Could you check a few things on this model? Use its own coordinates, in mm. Face numbers are marked on the shaded views. A direction names the side the tool comes from. Coordinates: 2 decimals unless noted, no trailing zeros. Order: outer loops, then holes, each group sorted by start corner. A loop starts at its lowest first (then second) coordinate and runs counter-clockwise, first axis right, second up. Notation, with made-up numbers: (28.5, 59) - (58.5, 59) arc R5 cw to (58.5, 66) - close; hole circle Ø1 at (18.25, -23). An arc over 180 degrees is marked (long way). Answer as CSV lines item,"result". Start each with the question number.
1. I want a section at C-C, the plane y = 0. Count the separate pieces of the cut face and the enclosed holes in it, and give its area (3 significant figures).
2. I want a section at D-D, the plane x = 9. List the corners of the cut face in (y, z) for me, and give its area (3 significant figures).
3. I need wall thicknesses on probe 1 along Z at (x, y) = (5, 4); probe 2 along Z at (x, y) = (2, 7); probe 3 along Y at (x, z) = (0.5, -1). Which ranges of each line are inside material? Lowest first, please.
4. Thinking about a two-plate mould opening in Y: for the marked faces 1, 2 and 3, which applies, released by +Y, released by -Y, zero draft, split by the parting line, or undercut?
5. I want a section at A-A, the plane x = 14.5. List the corners of the cut face in (y, z) for me, and give its area (3 significant figures).
6. For pin 1 (1.5 mm diameter, centred on x = 13, y = -12.5, fed in from -Z); pin 2 (2 mm diameter, centred on x = -10.5, z = 1.5, fed in from -Y); pin 3 (4 mm diameter, centred on x = 5.5, z = -0.5, fed in from -Y); pin 4 (3 mm diameter, centred on x = -9.9, y = -9.9, fed in from +Z), each with a flat end and sliding along its axis, tell me the tip position at first contact or that it passes through.
7. For the marked faces 4, 5 and 6, which set-ups out of +Z, -Z, +X, -X, +Y, -Y let a thin tool reach every point of the face, with its end or its side?
from build123d import *

# Parameters (mm, degrees)
SKETCH_1_R          = 17.5
EXTRUDE_1_DEPTH     = 2
SKETCH_2_R          = 7
EXTRUDE_2_DEPTH     = 7
SKETCH_3_R          = 17.5
EXTRUDE_3_DEPTH     = 2
SKETCH_4_W          = 5
SKETCH_4_H          = 5
CUT_EXTRUDE_1_DEPTH = 18
SKETCH_5_R          = 4.5
CUT_EXTRUDE_2_DEPTH = 18
SKETCH_6_R          = 6
SKETCH_6_R_2        = 4.5
EXTRUDE_4_DEPTH     = 2
SKETCH_7_R          = 2
CUT_EXTRUDE_3_DEPTH = 20
EXTRUDE_START       = 2
SKETCH_8_R          = 6
SKETCH_8_R_2        = 4.5
EXTRUDE_5_DEPTH     = 2
EXTRUDE_START_2     = 3
SKETCH_10_R         = 4.5
EXTRUDE_6_DEPTH     = 3


with BuildPart() as part:
    # 草图1 → 凸台-拉伸1 (new body)
    with BuildSketch(Plane.XY):
        Circle(SKETCH_1_R)
    extrude(amount=EXTRUDE_1_DEPTH)

    # 草图2 → 凸台-拉伸2 (add)
    with BuildSketch(Plane.XY.offset(2)):
        Circle(SKETCH_2_R)
    extrude(amount=EXTRUDE_2_DEPTH)

    # 草图3 → 凸台-拉伸3 (add)
    with BuildSketch(Plane.XY.offset(9)):
        Circle(SKETCH_3_R)
    extrude(amount=EXTRUDE_3_DEPTH)

    # 草图4 → 切除-拉伸1 (cut)
    with BuildSketch(Plane.XY.offset(11)):
        with Locations((-10.5, 0)):
            Rectangle(SKETCH_4_W, SKETCH_4_H)
    extrude(amount=-CUT_EXTRUDE_1_DEPTH, mode=Mode.SUBTRACT)

    # 草图5 → 切除-拉伸2 (cut)
    with BuildSketch(Plane(origin=(0, 0, 0), x_dir=(-1, 0, 0), z_dir=(0, 0, -1))):
        Circle(SKETCH_5_R)
    extrude(amount=-CUT_EXTRUDE_2_DEPTH, mode=Mode.SUBTRACT)

    # 草图6 → 凸台-拉伸4 (add)
    with BuildSketch(Plane.XY.offset(11)):
        Circle(SKETCH_6_R)
        with Locations(Location((0, 0, 0), (0, 0, 180))):
            Circle(SKETCH_6_R_2, mode=Mode.SUBTRACT)
    extrude(amount=EXTRUDE_4_DEPTH)

    # 草图7 → 切除-拉伸3 (cut)
    with BuildSketch(Plane.XY.offset(11)):
        with Locations((-9.899494937, 9.899494937)):
            Circle(SKETCH_7_R)
        with Locations((9.899494937, 9.899494937)):
            Circle(SKETCH_7_R)
        with Locations((9.899494937, -9.899494937)):
            Circle(SKETCH_7_R)
        with Locations((-9.899494937, -9.899494937)):
            Circle(SKETCH_7_R)
    extrude(amount=-CUT_EXTRUDE_3_DEPTH, mode=Mode.SUBTRACT)

    # 草图8 → 凸台-拉伸5 (add)
    with BuildSketch(Plane(origin=(0, 0, 0), x_dir=(-1, 0, 0), z_dir=(0, 0, -1)).offset(EXTRUDE_START)):
        with Locations(Location((0, 0, 0), (0, 0, 180))):
            Circle(SKETCH_8_R)
        Circle(SKETCH_8_R_2, mode=Mode.SUBTRACT)
    extrude(amount=-EXTRUDE_5_DEPTH)

    # 草图10 → 凸台-拉伸6 (add)
    with BuildSketch(Plane(origin=(0, 0, -2), x_dir=(-1, 0, 0), z_dir=(0, 0, -1)).offset(EXTRUDE_START_2)):
        Polygon((0, 8.082903769), (-7, 4.041451884), (-7, -4.041451884), (0, -8.082903769), (7, -4.041451884), (7, 4.041451884), align=None)
        Circle(SKETCH_10_R, mode=Mode.SUBTRACT)
    extrude(amount=-EXTRUDE_6_DEPTH)


solid = part.part
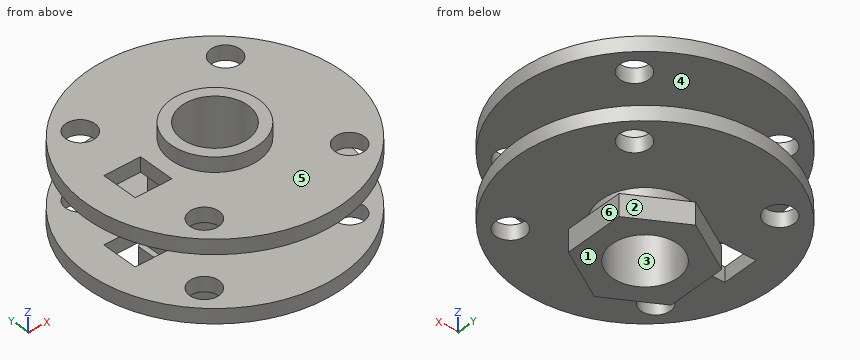
Solved:
1,separate pieces,"4"
1,enclosed holes,"0"
1,area,"146 mm2"
2,outline,"(-15.01, 0) - (-11.69, 0) - (-11.69, 2) - (-15.01, 2) - close; (-15.01, 9) - (-11.69, 9) - (-11.69, 11) - (-15.01, 11) - close; (-8.11, 0) - (8.11, 0) - (8.11, 2) - (-8.11, 2) - close; (-8.11, 9) - (8.11, 9) - (8.11, 11) - (-8.11, 11) - close; (11.69, 0) - (15.01, 0) - (15.01, 2) - (11.69, 2) - close; (11.69, 9) - (15.01, 9) - (15.01, 11) - (11.69, 11) - close"
2,area,"91.5 mm2"
3,probe 1,"z = -5 to -2, 0 to 11"
3,probe 2,"z = 0 to 2, 9 to 11"
3,probe 3,"y = -5.98 to -4.47, 4.47 to 5.98"
4,face 1,"zero draft"
4,face 2,"released by +Y"
4,face 3,"undercut"
5,outline,"(-9.8, 0) - (9.8, 0) - (9.8, 2) - (-9.8, 2) - close; (-9.8, 9) - (9.8, 9) - (9.8, 11) - (-9.8, 11) - close"
5,area,"78.4 mm2"
6,pin 1,"stops at z = 0"
6,pin 2,"stops at y = -14.7"
6,pin 3,"stops at y = -17.13"
6,pin 4,"passes through"
7,face 4,"none"
7,face 5,"+Z"
7,face 6,"-Z, +X, +Y, -Y"
